Study the drawing (mm; zero at the part's minimum x, y, z) and answer. A direction names the side the tool comes from. Coordinates: 2 decimals unless noted, no trailing zeros. Loops run counter-clockwise (first coordinate to the right, second up) from the corner with the lowest first, then second, coordinate; pieces in that order, holes last. Notation, with made-up numbers: (78.25, 55) - (107.25, 55) arc R27 cw to (107.25, 75) - close; hole circle Ø5 at (74.5, 52.5). An arc over 180 degrees is marked (long way). Use one line per item in the form item = value.
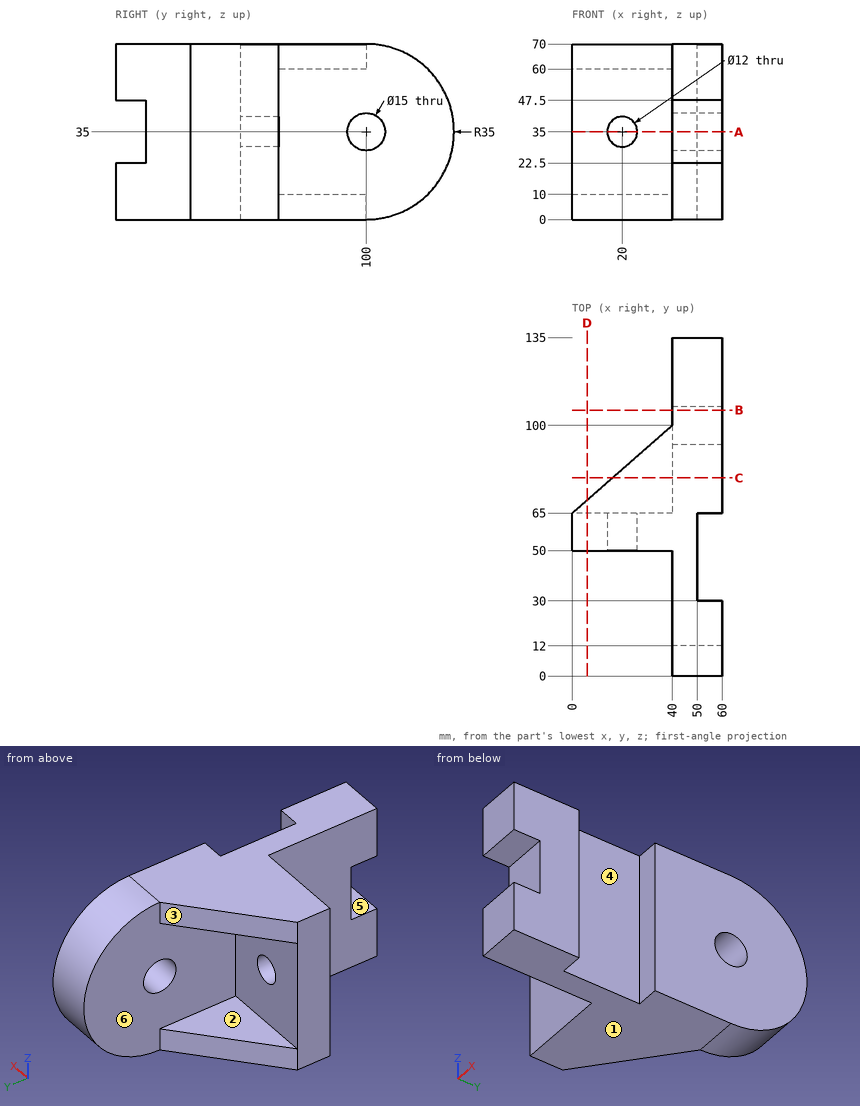
Item 1: Each of these flat-tipped pins is pushed along its axis until it touches: P1, Ø4, axis at x = 13.5, z = 63, coming from the -Y side; P2, Ø11, axis at x = 53.5, z = 41.5, coming from the -Y side; P3, Ø3, axis at x = 53.5, z = 33, coming from the +Y side. Where does it stop, or does it pass through?
Results below:
P1 = 50
P2 = 12
P3 = 135
Item 2: The part is cut by section D-D on x = 6. Give the vertices of the cut face in (y, z), plus the area to 4 significant figures.
Results below:
outline = (50, 0) - (70.25, 0) - (70.25, 10) - (65, 10) - (65, 60) - (70.25, 60) - (70.25, 70) - (50, 70) - close
area = 1,155 mm²
Item 3: Find the intervals of material crossed by L1, parallel to Z at x = 46.5, y = 100; L2, parallel to Z at x = 24, y = 82; L3, parallel to X at y = 92, z = 59, in increasing order.
Results below:
L1 = 0 to 27.5, 42.5 to 70
L2 = 0 to 10, 60 to 70
L3 = 40 to 60
Item 4: The part is cut by section C-C on y = 79. Give the vertices of the cut face in (x, z), plus the area to 3 significant figures.
Results below:
outline = (16, 0) - (60, 0) - (60, 70) - (16, 70) - (16, 60) - (40, 60) - (40, 10) - (16, 10) - close
area = 1,880 mm²
Item 5: Which of the six approach directions +Z, -Z, +X, -X, +Y, -Y give full straight-line access (tool end or side, diameter ignored) to the marked faces 4, 5 and 6?
Results below:
face_4 = +Z, -Z, +X
face_5 = +X, -X, -Y
face_6 = -X, +Y
Item 6: The part is cut by section A-A on z = 35. Give the vertices of the cut face in (x, y).
Results below:
outline = (0, 50) - (14, 50) - (14, 65) - (0, 65) - close; (26, 50) - (40, 50) - (40, 12) - (60, 12) - (60, 30) - (50, 30) - (50, 65) - (60, 65) - (60, 92.5) - (40, 92.5) - (40, 65) - (26, 65) - close; (40, 107.5) - (60, 107.5) - (60, 135) - (40, 135) - close
Item 7: The part is cut by section B-B on y = 106. Give the vertices of the cut face in (x, z).
Results below:
outline = (40, 0.52) - (60, 0.52) - (60, 30.5) - (40, 30.5) - close; (40, 39.5) - (60, 39.5) - (60, 69.48) - (40, 69.48) - close
Item 8: For a pull along Z with two mould halves and no side action, classify the marked faces 1, 2 and 3 as +Z half, -Z half, draft (parallel to the pull), parting line (faces both ways), or undercut.
Results below:
face_1 = -Z half
face_2 = undercut
face_3 = draft
